For this review, take the finished solid that the model builds, in its own axes (mm). A direction names the side the tool comes from. Coordinates: 2 decimals unless noted, no trailing zeros. Loops run counter-clockwise (first coordinate to the right, second up) from the corner with the lowest first, then second, coordinate; pieces in that order, holes last. Notation, with made-up numbers: M -19.5,11.5 L -11.5,11.5 A17 ccw -11.5,33.5 Z; hole C 28.5,82 d10. An arc over 180 degrees is marked long. Answer as a JSON object with one key per item and string values. Group by question number.
Item 1: Mouldability with a two-part tool opening along Y and no side actions: class faces 1 (the face through (236.978, 15.755, 1.479)), 2 (the face through (276.216, 5.321, 1.479)), 3 (the face through (279.068, 50, 1)), 4 (the face through (136.92, 94.306, 1.479)) as +Y half, -Y half, draft (parallel to the pull), parting line (faces both ways), or undercut.
Item 2: Wall thickness on L1, parallel to X at y = 71, z = 0.15; L2, parallel to Y at x = 253.5, z = 1.75; L3, parallel to X at y = 37, z = 0.2: over which ranges is each line inside the solid? List them lowest first. Write a range as from..to.
Item 3: Add section C-C (z = 0.75). Count the separate pieces of the cut face and the enclosed holes in it, then the cut area to 3 significant figures.
Item 4: Tool access review of faces 5 (the face through (237.08, 83.98, 1.48)), 6 (the face through (276.06, 94.46, 1.48)): name each direction out of +Z, -Z, +X, -X, +Y, -Y from which nothing blocks a thin tool from reaching the whole face with its end or side.
Item 5: Insertion check: pin 1 (2.5 mm diameter, centred on x = 177.57, y = 18.03, fed in from -Z). The pin has a flat end and moves straight along its axis. Give the tip position at first contact, or say it passes through.
Item 6: Add section A-A (x = 226). State the section outline as (y, z) points, then the cut area to 3 significant figures.
Item 7: Add section B-B (y = 64). State the section outline as (x, z) points.
from build123d import *

# Parameters (mm, degrees)
SKETCH_1_R          = 1.5
EXTRUDE_1_DEPTH     = 3
SKETCH_2_R          = 1.6
CUT_EXTRUDE_1_DEPTH = 296.563476419


with BuildPart() as part:
    # 草图1 → 凸台-拉伸1 (new body)
    with BuildSketch(Plane(origin=(0, 0, 0), x_dir=(-1, 0, 0), z_dir=(0, 0, -1))):
        with BuildLine():
            Line((-269.068, 2.31372), (-144.068, 2.31372))
            ThreePointArc((-144.068, 2.31372), (-136.996932188, 5.242652188), (-134.068, 12.31372))
            Line((-134.068, 12.31372), (-134.068, 87.313))
            ThreePointArc((-134.068, 87.313), (-136.996932188, 94.384067812), (-144.068, 97.313))
            Line((-144.068, 97.313), (-269.068, 97.313))
            ThreePointArc((-269.068, 97.313), (-276.139067812, 94.384067812), (-279.068, 87.313))
            Line((-279.068, 87.313), (-279.068, 12.31372))
            ThreePointArc((-279.068, 12.31372), (-276.139067812, 5.242652188), (-269.068, 2.31372))
        make_face()
        with Locations(Location((-144.568, 70.12826533, 0), (0, 0, 180))):
            Circle(SKETCH_1_R, mode=Mode.SUBTRACT)
        with Locations(Location((-192.767, 68.82896533, 0), (0, 0, 180))):
            Circle(SKETCH_1_R, mode=Mode.SUBTRACT)
        with Locations(Location((-149.668, 18.02876533, 0), (0, 0, 180))):
            Circle(SKETCH_1_R, mode=Mode.SUBTRACT)
        with Locations(Location((-215.068, 71.68966533, 0), (0, 0, 180))):
            Circle(SKETCH_1_R, mode=Mode.SUBTRACT)
        with Locations(Location((-259.067, 71.68966533, 0), (0, 0, 180))):
            Circle(SKETCH_1_R, mode=Mode.SUBTRACT)
        with Locations(Location((-259.067, 27.68886533, 0), (0, 0, 180))):
            Circle(SKETCH_1_R, mode=Mode.SUBTRACT)
        with Locations(Location((-215.068, 27.68886533, 0), (0, 0, 180))):
            Circle(SKETCH_1_R, mode=Mode.SUBTRACT)
        with Locations(Location((-177.568, 18.02876533, 0), (0, 0, 180))):
            Circle(SKETCH_1_R, mode=Mode.SUBTRACT)
        with BuildLine():
            Line((-270.266244411, 51.969241805), (-239.172302587, 83.100283559))
            ThreePointArc((-239.172302587, 83.100283559), (-237.051506509, 83.980227838), (-234.929662654, 83.102813116))
            Line((-234.929662654, 83.102813116), (-203.798358898, 52.008609603))
            ThreePointArc((-203.798358898, 52.008609603), (-202.918414619, 49.887813524), (-203.795829341, 47.765969669))
            Line((-203.795829341, 47.765969669), (-234.889771164, 16.634927916))
            ThreePointArc((-234.889771164, 16.634927916), (-237.010567242, 15.754983637), (-239.132411097, 16.632398358))
            Line((-239.132411097, 16.632398358), (-270.263714853, 47.726601872))
            ThreePointArc((-270.263714853, 47.726601872), (-271.143659132, 49.84739795), (-270.266244411, 51.969241805))
        make_face(mode=Mode.SUBTRACT)
    extrude(amount=-EXTRUDE_1_DEPTH)

    # 草图2 → 切除-拉伸1 (cut, through all)
    with BuildSketch(Plane.XY.offset(3)):
        with Locations((259.067, 71.68966533)):
            Circle(SKETCH_2_R)
        with Locations((215.068, 71.68966533)):
            Circle(SKETCH_2_R)
        with Locations((215.068, 27.68886533)):
            Circle(SKETCH_2_R)
        with Locations((259.067, 27.68886533)):
            Circle(SKETCH_2_R)
    extrude(amount=-CUT_EXTRUDE_1_DEPTH, mode=Mode.SUBTRACT)


solid = part.part
From the geometry:
{
 "1": {"face 1": "undercut", "face 2": "-Y half", "face 3": "draft", "face 4": "+Y half"},
 "2": {"L1": "x = 134.07..143.35, 145.79..213.62, 216.51..222.81, 251.26..257.62, 260.51..279.07", "L2": "y = 2.31..30.98, 68.76..97.31", "L3": "x = 134.07..214.55, 259.52..279.07"},
 "3": {"separate pieces": "1", "enclosed holes": "9", "area": "11,100 mm²"},
 "4": {"face 5": "+Z, -Z", "face 6": "+Z, -Z, +X, +Y"},
 "5": {"pin 1": "passes through"},
 "6": {"outline": "M 2.31,0 L 25.54,0 L 25.54,3 L 2.31,3 Z; M 74.18,0 L 97.31,0 L 97.31,3 L 74.18,3 Z", "area": "139 mm²"},
 "7": {"outline": "M 134.07,0 L 215.8,0 L 215.8,3 L 134.07,3 Z; M 258.25,0 L 279.07,0 L 279.07,3 L 258.25,3 Z"}
}
